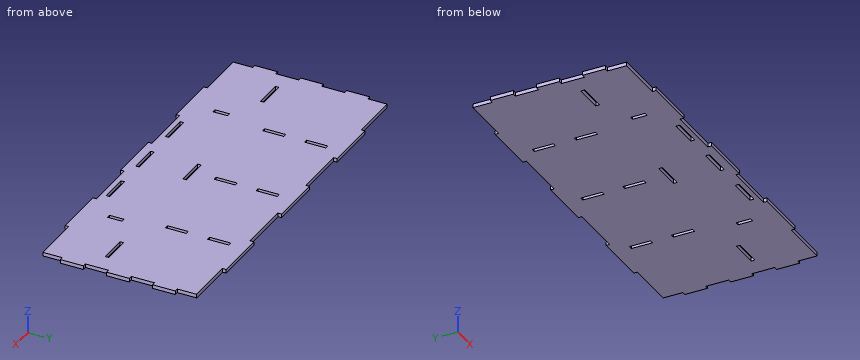
Autodesk Inventor part; units mm, degrees
ref_plane "YZ Plane" through (0, 0, 0) normal (1, 0, 0) x (0, 1, 0)
ref_plane "XZ Plane" through (0, 0, 0) normal (0, 1, 0) x (-1, 0, 0)
ref_plane "XY Plane" through (0, 0, 0) normal (0, 0, 1) x (1, 0, 0)
sketch "Sketch1" plane through (0, 0, 0) normal (0, 0, 1) x (1, 0, 0)
  line L0 (-150, 18.5714) -> (-147, 18.5714)
  line L1 (-147, 37.1429) -> (-150, 37.1429)
  line L2 (-150, 55.7143) -> (-147, 55.7143)
  line L3 (-147, 74.2857) -> (-150, 74.2857)
  line L4 (-150, 92.8571) -> (-147, 92.8571)
  line L5 (-147, 111.4286) -> (-150, 111.4286)
  line L6 (147, 18.5714) -> (150, 18.5714)
  line L7 (147, 37.1429) -> (150, 37.1429)
  line L8 (150, 55.7143) -> (147, 55.7143)
  line L9 (147, 74.2857) -> (150, 74.2857)
  line L10 (150, 92.8571) -> (147, 92.8571)
  line L11 (150, 111.4286) -> (147, 111.4286)
  line L12 (-107.1429, 0) -> (-107.1429, 3)
  line L13 (-64.2857, 3) -> (-64.2857, 0)
  line L14 (-21.4286, 0) -> (-21.4286, 3)
  line L15 (21.4286, 0) -> (21.4286, 3)
  line L16 (64.2857, 0) -> (64.2857, 3)
  line L17 (107.1429, 0) -> (107.1429, 3)
  line L18 (-107.1429, 127) -> (-107.1429, 130)
  line L19 (-64.2857, 127) -> (-64.2857, 130)
  line L20 (-21.4286, 127) -> (-21.4286, 130)
  line L21 (21.4286, 127) -> (21.4286, 130)
  line L22 (64.2857, 127) -> (64.2857, 130)
  line L23 (107.1429, 127) -> (107.1429, 130)
  line L24 (-107.1429, 3) -> (-147, 3)
  line L25 (-147, 3) -> (-147, 18.5714)
  line L26 (-147, 37.1429) -> (-147, 55.7143)
  line L27 (-147, 74.2857) -> (-147, 92.8571)
  line L28 (-147, 111.4286) -> (-147, 127)
  line L29 (-147, 127) -> (-107.1429, 127)
  line L30 (-64.2857, 127) -> (-21.4286, 127)
  line L31 (21.4286, 127) -> (64.2857, 127)
  line L32 (107.1429, 127) -> (147, 127)
  line L33 (-21.4286, 3) -> (-64.2857, 3)
  line L34 (147, 3) -> (107.1429, 3)
  line L35 (64.2857, 3) -> (21.4286, 3)
  line L36 (-150, 92.8571) -> (-150, 111.4286)
  line L37 (-150, 18.5714) -> (-150, 37.1429)
  line L38 (-150, 55.7143) -> (-150, 74.2857)
  line L39 (-64.2857, 0) -> (-107.1429, 0)
  line L40 (107.1429, 0) -> (64.2857, 0)
  line L41 (21.4286, 0) -> (-21.4286, 0)
  line L42 (-107.1429, 130) -> (-64.2857, 130)
  line L43 (-21.4286, 130) -> (21.4286, 130)
  line L44 (64.2857, 130) -> (107.1429, 130)
  line L45 (150, 37.1429) -> (150, 18.5714)
  line L46 (150, 111.4286) -> (150, 92.8571)
  line L47 (150, 74.2857) -> (150, 55.7143)
  line L48 (147, 127) -> (147, 111.4286)
  line L49 (147, 92.8571) -> (147, 74.2857)
  line L50 (147, 55.7143) -> (147, 37.1429)
  line L51 (147, 18.5714) -> (147, 3)
  point P0 (0, 0)
  dimension "d1" = 300
  dimension "d5" = 42.8571
  dimension "d6" = 150
  dimension "d7" = 85.7143
  dimension "d8" = 128.5714
  dimension "d9" = 171.4286
  dimension "d10" = 214.2857
  dimension "d11" = 257.1429
  dimension "d12" = 130
  dimension "d13" = 18.5714
  dimension "d14" = 0
  dimension "d15" = 3
  dimension "d16" = 37.1429
  dimension "d17" = 55.7143
  dimension "d18" = 74.2857
  dimension "d19" = 92.8571
  dimension "d20" = 111.4286
  dimension "d21" = 124
  dimension "d22" = 3
  dimension "d23" = 3
extrude "Extrusion1" add sketch "Sketch1" along normal blind 3
sketch "Sketch2" plane through (0, 0, 3) normal (0, 0, 1) x (1, 0, 0)
  line L0 (-108.5714, 45) -> (-131.4286, 45)
  line L1 (-131.4286, 45) -> (-131.4286, 48)
  line L2 (-131.4286, 48) -> (-108.5714, 48)
  line L3 (-108.5714, 48) -> (-108.5714, 45)
  line L4 (-11.4286, 45) -> (11.4286, 45)
  line L5 (11.4286, 45) -> (11.4286, 48)
  line L6 (11.4286, 48) -> (-11.4286, 48)
  line L7 (-11.4286, 48) -> (-11.4286, 45)
  line L8 (108.5714, 45) -> (131.4286, 45)
  line L9 (131.4286, 45) -> (131.4286, 48)
  line L10 (131.4286, 48) -> (108.5714, 48)
  line L11 (108.5714, 48) -> (108.5714, 45)
  line L12 (-21.4286, 0) -> (21.4286, 0)
  line L13 (-11.4286, 10) -> (11.4286, 10)
  line L14 (11.4286, 10) -> (11.4286, 7)
  line L15 (11.4286, 7) -> (-11.4286, 7)
  line L16 (-11.4286, 7) -> (-11.4286, 10)
  line L17 (34.2857, 7) -> (57.1429, 7)
  line L18 (57.1429, 7) -> (57.1429, 10)
  line L19 (57.1429, 10) -> (34.2857, 10)
  line L20 (34.2857, 10) -> (34.2857, 7)
  line L21 (-34.2857, 7) -> (-57.1429, 7)
  line L22 (-57.1429, 7) -> (-57.1429, 10)
  line L23 (-57.1429, 10) -> (-34.2857, 10)
  line L24 (-34.2857, 10) -> (-34.2857, 7)
  line L25 (-80, 21.6667) -> (-83, 21.6667)
  line L26 (-83, 21.6667) -> (-83, 33.3333)
  line L27 (-83, 33.3333) -> (-80, 33.3333)
  line L28 (-80, 33.3333) -> (-80, 21.6667)
  line L29 (80, 21.6667) -> (83, 21.6667)
  line L30 (83, 21.6667) -> (83, 33.3333)
  line L31 (83, 33.3333) -> (80, 33.3333)
  line L32 (80, 33.3333) -> (80, 21.6667)
  point P0 (0, 0)
  point P1 (-120, 45)
  point P2 (120, 45)
  dimension "d26" = 22.8571
  dimension "d27" = 48
  dimension "d28" = 3
  dimension "d29" = 120
  dimension "d30" = 120
  dimension "d31" = 11.4286
  dimension "d34" = 7
  dimension "d35" = 3
  dimension "d36" = 22.8571
  dimension "d37" = 22.8571
  dimension "d38" = 3
  dimension "d39" = 3
  dimension "d40" = 11.6667
  dimension "d41" = 11.6667
  dimension "d42" = 22.8571
  dimension "d43" = 22.8571
extrude "Extrusion2" cut sketch "Sketch2" against normal through all
sketch "Sketch3" plane through (0, 0, 3) normal (0, 0, 1) x (1, 0, 0)
  line L0 (-76.5, 116) -> (-73.5, 116)
  line L1 (-73.5, 116) -> (-73.5, 99)
  line L2 (-73.5, 99) -> (-76.5, 99)
  line L3 (-76.5, 99) -> (-76.5, 116)
  line L4 (-76.5, 82) -> (-73.5, 82)
  line L5 (-73.5, 82) -> (-73.5, 65)
  line L6 (-73.5, 65) -> (-76.5, 65)
  line L7 (-76.5, 65) -> (-76.5, 82)
  line L8 (-21.4286, 127) -> (-64.2857, 127)
  line L9 (-64.2857, 127) -> (-73.5, 127) construction
  line L10 (-73.5, 127) -> (-73.5, 116) construction
  line L11 (-73.5, 99) -> (-73.5, 82) construction
  line L12 (-108.5714, 48) -> (-73.5, 48) construction
  line L13 (-73.5, 48) -> (-73.5, 65) construction
  point P0 (0, 0)
  dimension "d44" = 17
  dimension "d45" = 3
  dimension "d46" = 73.5
  dimension "d52" = 17
extrude "Extrusion3" cut sketch "Sketch3" against normal through all
pattern_linear "Rectangular Pattern1" count 3 spacing 75 along (1, 0, 0) of "Extrusion3"
equation "\"d1\" = wt"
equation "\"d5\" = 0.142857 * wt - tol"
equation "\"d7\" = 0.285714 * wt + tol"
equation "\"d8\" = 0.428571 * wt - tol"
equation "\"d9\" = 0.571429 * wt + tol"
equation "\"d10\" = 0.714286 * wt - tol"
equation "\"d11\" = 0.857143 * wt + tol"
equation "\"d13\" = 0.142857 * height_back - tol"
equation "\"d15\" = tt"
equation "\"d16\" = 0.285714 * height_back + tol"
equation "\"d17\" = 0.428571 * height_back - tol"
equation "\"d18\" = 0.571429 * height_back + tol"
equation "\"d19\" = 0.714286 * height_back - tol"
equation "\"d20\" = 0.857143 * height_back + tol"
equation "\"d21\" = -2 * tt + height_back"
equation "\"d22\" = tt"
equation "\"d23\" = tt"
equation "\"d24\" = tt"
equation "\"d26\" = 0.142857 * shelfW + 2 * tol"
equation "\"d28\" = tt"
equation "\"d35\" = tt"
equation "\"d36\" = 0.142857 * shelfW - 2 * tol"
equation "\"d37\" = 0.142857 * shelfW - 2 * tol"
equation "\"d38\" = tt"
equation "\"d39\" = tt"
equation "\"d40\" = 0.333333 * shelfH + 2 * tol"
equation "\"d41\" = 0.333333 * shelfH - tol"
equation "\"d42\" = 0.142857 * shelfW - tol"
equation "\"d43\" = 0.142857 * shelfW - tol"
equation "\"d45\" = tt"
equation "\"d51\" = 0.25 * wt"
equation "\"wt\" = 300"
equation "\"tt\" = 3"
equation "\"tol\" = 0"
equation "\"height_back\" = 130"
equation "\"d4\" = tt"
equation "\"tiroir\" = 1"
equation "\"nHoles\" = 4"
equation "\"shelfH\" = 35"
properties part number "back"
Check sheet for the modelled part. Datum: model origin and axes. Units: mm. Round coordinates to 2 decimals unless told otherwise and drop trailing zeros. Order: outer loops, then holes, each group sorted by start corner. A loop starts at its lowest first (then second) coordinate and runs counter-clockwise, first axis right, second up.
1) Scan lines: line 1 (X direction, y = 31, z = 1.9); line 2 (X direction, y = 46, z = 2.6); line 3 (X direction, y = 9.5, z = 1.4). Record each from-to range of solid material in increasing order.
2) Section check D-D (y = 13). Record the boundary of the cut face in (x, z), and give its area (3 significant figures).
3) Section check A-A (y = 28.5). Record the boundary of the cut face in (x, z).
4) Section check C-C (z = 0.8). Give the number of separate pieces and of enclosed holes in the cut face, and give its area (3 significant figures).
5) Go/stop test with flat-tipped pins: pin 1 Ø6 at (x, y) = (83, 92) entering from -Z; pin 2 Ø0.9 at (x, z) = (-135, 1) entering from +Y. Record where each tip stops, or that it passes through.
6) Section check B-B (x = 41.5). Record the boundary of the cut face in (y, z), and give its area (3 significant figures).
Result:
1. line 1: x = -150 to -83, -80 to 80, 83 to 150
1. line 2: x = -147 to -131.43, -108.57 to -11.43, 11.43 to 108.57, 131.43 to 147
1. line 3: x = -147 to -57.14, -34.29 to -11.43, 11.43 to 34.29, 57.14 to 147
2. outline: (-147, 0) - (147, 0) - (147, 3) - (-147, 3) - close
2. area: 882 mm2
3. outline: (-150, 0) - (-83, 0) - (-83, 3) - (-150, 3) - close; (-80, 0) - (80, 0) - (80, 3) - (-80, 3) - close; (83, 0) - (150, 0) - (150, 3) - (83, 3) - close
4. separate pieces: 1
4. enclosed holes: 14
4. area: 36,800 mm2
5. pin 1: stops at z = 0
5. pin 2: stops at y = 127
6. outline: (3, 0) - (7, 0) - (7, 3) - (3, 3) - close; (10, 0) - (127, 0) - (127, 3) - (10, 3) - close
6. area: 363 mm2
